Read the model definition and answer for the solid it produces. Units are mm, in the model's axes. Coordinates: 2 decimals unless noted, no trailing zeros. Loops run counter-clockwise (first coordinate to the right, second up) from the corner with the lowest first, then second, coordinate; pieces in that order, holes last.
Autodesk Inventor part; units mm, degrees
ref_plane "YZ Plane" through (0, 0, 0) normal (1, 0, 0) x (0, 1, 0)
ref_plane "XZ Plane" through (0, 0, 0) normal (0, 1, 0) x (-1, 0, 0)
ref_plane "XY Plane" through (0, 0, 0) normal (0, 0, 1) x (1, 0, 0)
sketch "Sketch1" plane through (0, 0, 0) normal (0, 0, 1) x (1, 0, 0)
  line L0 (95, 60) -> (105, 60)
  line L1 (105, 60) -> (105, 10)
  line L2 (105, 10) -> (100, 10)
  line L3 (100, 10) -> (100, 20)
  line L4 (100, 20) -> (95, 20)
  line L5 (95, 20) -> (95, 60)
  line L6 (105, -60) -> (95, -60)
  line L7 (95, -60) -> (95, -20)
  line L8 (95, -20) -> (100, -20)
  line L9 (100, -20) -> (100, -10)
  line L10 (100, -10) -> (105, -10)
  line L11 (105, -10) -> (105, -60)
  line L12 (120.5, 3.5) -> (123.5, 3.5)
  line L13 (123.5, 3.5) -> (123.5, 5)
  line L14 (123.5, 5) -> (127, 5)
  line L15 (127, 5) -> (127, -5)
  line L16 (127, -5) -> (123.5, -5)
  line L17 (123.5, -5) -> (123.5, -3.5)
  line L18 (123.5, -3.5) -> (120.5, -3.5)
  line L19 (120.5, -3.5) -> (120.5, -5)
  line L20 (120.5, -5) -> (117, -5)
  line L21 (117, -5) -> (117, -49)
  line L22 (117, -49) -> (107, -51)
  line L23 (107, -51) -> (107, -10)
  line L24 (107, -10) -> (112, -10)
  line L25 (112, -10) -> (112, -3.5)
  line L26 (112, -3.5) -> (100, -3.5)
  line L27 (100, -3.5) -> (100, -4)
  line L28 (100, -4) -> (45, -4)
  arc A0 (43, -6) -> (45, -4) centre (43, -4) ccw
  line L29 (43, -6) -> (42, -6)
  arc A1 (40, -4) -> (42, -6) centre (42, -4) ccw
  line L30 (40, -4) -> (5, -4)
  arc A2 (3, -6) -> (5, -4) centre (3, -4) ccw
  line L31 (3, -6) -> (2, -6)
  arc A3 (0, -4) -> (2, -6) centre (2, -4) ccw
  line L32 (0, -4) -> (0, 4)
  arc A4 (2, 6) -> (0, 4) centre (2, 4) ccw
  line L33 (2, 6) -> (3, 6)
  arc A5 (5, 4) -> (3, 6) centre (3, 4) ccw
  line L34 (5, 4) -> (40, 4)
  arc A6 (42, 6) -> (40, 4) centre (42, 4) ccw
  line L35 (42, 6) -> (43, 6)
  arc A7 (45, 4) -> (43, 6) centre (43, 4) ccw
  line L36 (45, 4) -> (100, 4)
  line L37 (100, 4) -> (100, 3.5)
  line L38 (100, 3.5) -> (112, 3.5)
  line L39 (112, 3.5) -> (112, 10)
  line L40 (112, 10) -> (107, 10)
  line L41 (107, 10) -> (107, 51)
  line L42 (107, 51) -> (117, 49)
  line L43 (117, 49) -> (117, 5)
  line L44 (117, 5) -> (120.5, 5)
  line L45 (120.5, 5) -> (120.5, 3.5)
  line L46 (92, 27.5) -> (92, 26)
  line L47 (92, 26) -> (42, 26)
  line L48 (42, 26) -> (42, 27.5)
  line L49 (42, 27.5) -> (92, 27.5)
  line L50 (92, -24) -> (92, -25.5)
  line L51 (92, -25.5) -> (42, -25.5)
  line L52 (42, -25.5) -> (42, -24)
  line L53 (42, -24) -> (92, -24)
  line L54 (92, -25.5) -> (82, -25.5)
  line L55 (82, -25.5) -> (82, -24)
  line L56 (82, -24) -> (77, -24)
  line L57 (77, -24) -> (77, -25.5)
  line L58 (77, -25.5) -> (57, -25.5)
  line L59 (57, -25.5) -> (57, -24)
  line L60 (57, -24) -> (52, -24)
  line L61 (52, -24) -> (52, -25.5)
  line L62 (52, -25.5) -> (42, -25.5)
  line L63 (42, -25.5) -> (42, 27.5)
  line L64 (92, 27.5) -> (92, 97.5)
  line L65 (92, -25.5) -> (92, -65.5)
  line L66 (92, -65.5) -> (132, -65.5)
  line L67 (132, -65.5) -> (142, -65.5)
  line L68 (132, -65.5) -> (132, 97.5)
  line L69 (142, -65.5) -> (142, 109.5)
  line L70 (42, 27.5) -> (34, 27.5)
  line L71 (95, 60) -> (105, 60)
  line L72 (105, 60) -> (105, 84)
  line L73 (105, 84) -> (95, 84)
  line L74 (95, 84) -> (95, 60)
  line L75 (95, 60) -> (95, 90)
  line L76 (95, 90) -> (132, 90)
  line L77 (95, 90) -> (92, 90)
  line L78 (142, -65.5) -> (142, -95.5)
  line L79 (142, -95.5) -> (92, -95.5)
  line L80 (92, -95.5) -> (34, -25.5)
  line L81 (34, -25.5) -> (34, 27.5)
  line L82 (0, 0) -> (71, 0)
  line L83 (23.8389, -219.7015) -> (66.8389, -219.7015)
  line L84 (66.8389, -219.7015) -> (66.8389, -198.7015)
  line L85 (66.8389, -198.7015) -> (23.8389, -198.7015)
  line L86 (23.8389, -198.7015) -> (23.8389, -219.7015)
  line L87 (45.3389, -198.7015) -> (45.3389, -219.7015)
  line L88 (66.8389, -198.7015) -> (66.8389, -203.7015)
  line L89 (66.8389, -203.7015) -> (70.8389, -203.7015)
  line L90 (70.8389, -203.7015) -> (70.8389, -213.7015)
  circle A8 centre (70.8389, -213.7015) radius 2
  circle A9 centre (70.8389, -203.7015) radius 2
  line L91 (66.8389, -209.2015) -> (56.8389, -209.2015)
  line L92 (56.8389, -209.2015) -> (56.8389, -189.2015)
  line L93 (56.8389, -189.2015) -> (56.8389, -229.2015)
  circle A10 centre (19.8389, -213.7015) radius 2
  circle A11 centre (19.8389, -203.7015) radius 2
  line L94 (33.8389, -189.2015) -> (33.8389, -229.2015)
  line L95 (42, -24) -> (83, -24)
  line L96 (83, -24) -> (83, -4)
  line L97 (83, -4) -> (42, -4)
  line L98 (42, -4) -> (42, -24)
  line L99 (62.5, -4) -> (62.5, -24)
  line L100 (83, -4) -> (83, -9)
  line L101 (83, -9) -> (87, -9)
  line L102 (87, -9) -> (87, -19)
  circle A12 centre (87, -9) radius 2
  circle A13 centre (87, -19) radius 2
  circle A14 centre (38, -9) radius 2
  circle A15 centre (38, -19) radius 2
  line L103 (92, -24) -> (92, 26)
  line L104 (109.5, -120.7576) -> (69.5, -120.7576)
  line L105 (69.5, -120.7576) -> (69.5, 125.4146)
  line L106 (142, 109.5) -> (67, 109.5)
  line L107 (67, 109.5) -> (67, 109.5)
  line L108 (67, 109.5) -> (34, 27.5)
  line L109 (34, 27.5) -> (69.5, 27.5)
  line L110 (69.5, 27.5) -> (69.5, 52.5)
  line L111 (92, 27.5) -> (69.5, 27.5)
  line L112 (92, 27.5) -> (77, 27.5)
  line L113 (77, 27.5) -> (77, 52.5)
  line L114 (77, 52.5) -> (78.5, 52.5)
  line L115 (78.5, 72.5) -> (77, 72.5)
  line L116 (77, 72.5) -> (77, 52.5)
  line L117 (78.5, 52.5) -> (81, 52.5)
  line L118 (81, 52.5) -> (81, 72.5)
  line L119 (81, 72.5) -> (78.5, 72.5)
  line L120 (81, 62.5) -> (79, 62.5)
  line L121 (79, 62.5) -> (74, 62.5)
  line L122 (74, 62.5) -> (84, 62.5)
  circle A16 centre (74, 62.5) radius 1.5
  circle A17 centre (84, 62.5) radius 1.5
  line L123 (92, -95.5) -> (92, -90.5)
  line L124 (92, -90.5) -> (97, -90.5)
  line L125 (97, -90.5) -> (117, -90.5)
  line L126 (117, -90.5) -> (117, -89)
  line L127 (117, -89) -> (97, -89)
  line L128 (97, -89) -> (97, -90.5)
  line L129 (97, -89) -> (97, -79)
  line L130 (97, -79) -> (117, -79)
  line L131 (117, -79) -> (117, -77.5)
  line L132 (117, -77.5) -> (97, -77.5)
  line L133 (97, -77.5) -> (97, -79)
  line L134 (107, -90.5) -> (107, -84)
  circle A18 centre (107, -84) radius 1.5
  point P0 (59.5188, -93.2152)
  point P1 (83, -4)
  point P2 (83, -24)
  dimension "d0" = 10
  dimension "d1" = 1.5
  dimension "d2" = 5
  dimension "d3" = 1.5
  dimension "d4" = 20
  dimension "d5" = 1.5
  dimension "d6" = 5
  dimension "d7" = 1.5
  dimension "d8" = 70
  dimension "d9" = 40
  dimension "d10" = 40
  dimension "d11" = 40
  dimension "d12" = 10
  dimension "d13" = 175
  dimension "d14" = 8
  dimension "d15" = 10
  dimension "d16" = 24
  dimension "d17" = 30
  dimension "d19" = 30
  dimension "d20" = 50
  dimension "d21" = 71
  dimension "d22" = 43
  dimension "d23" = 21
  dimension "d24" = 5
  dimension "d25" = 4
  dimension "d26" = 10
  dimension "d27" = 4
  dimension "d28" = 4
  dimension "d29" = 10
  dimension "d30" = 20
  dimension "d31" = 40
  dimension "d32" = 41
  dimension "d33" = 20
  dimension "d34" = 5
  dimension "d35" = 4
  dimension "d36" = 10
  dimension "d37" = 4
  dimension "d38" = 4
  dimension "d48" = 40
  dimension "d49" = 3
  dimension "d50" = 75
  dimension "d51" = 0
  dimension "d62" = 15
  dimension "d63" = 25
  dimension "d64" = 1.5
  dimension "d65" = 20
  dimension "d73" = 2.5
  dimension "d74" = 2
  dimension "d75" = 5
  dimension "d76" = 10
  dimension "d77" = 3
  dimension "d78" = 3
  dimension "d81" = 5
  dimension "d82" = 5
  dimension "d83" = 20
  dimension "d84" = 1.5
  dimension "d85" = 10
  dimension "d86" = 20
  dimension "d87" = 1.5
  dimension "d88" = 3
extrude "Extrusion1" add sketch "Sketch1" along normal blind 1.5 contours A16 | A17 | L116 L121 L120 L118 L117 L114 | L77 L64 L49 L105 L106 L69 L67 L68 L76 | L133 L132 L131 L130 | A18 | L128 L127 L134 L125 | L67 L78 L79 L80 L105 L51 L65 L66 | L103 L36 L105 L47 | L105 L36 A7 L35 L63 L47 | L103 L28 L105 L36 | L49 L70 L108 L106 L105 | L53 L96 L28 L103 | L63 A6 L34 L81 L70 L48 | L105 L82 L63 L35 A7 L36 | L116 L115 L119 L118 L120 L121 | L80 L81 L30 A1 L63 L52 L51 L105 | L63 L82 L81 L34 A6 | L105 L28 L97 L63 L82 | L63 A1 L30 L81 L82 | L134 L127 L126 L125
sketch "Sketch2" plane through (0, 0, 1.5) normal (0, 0, 1) x (1, 0, 0)
  line L0 (42, 26) -> (42, 27.5)
  line L1 (42, 26.75) -> (62, 26.75)
  line L2 (62, 26.75) -> (62, 31.75)
  line L3 (62, 31.75) -> (62, 21.75)
  circle A0 centre (62, 31.75) radius 1.5
  circle A1 centre (62, 21.75) radius 1.5
  point P0 (0, 0)
  dimension "d41" = 20
  dimension "d42" = 5
  dimension "d43" = 10
  dimension "d44" = 3
  dimension "d45" = 3
extrude "Extrusion2" cut sketch "Sketch2" against normal blind 1.5
extrude "Extrusion5" cut sketch "Sketch1" along normal blind 1.5 contours A16 | A17 | L116 L121 L120 L118 L117 L114 | L116 L115 L119 L118 L120 L121
extrude "Extrusion6" cut sketch "Sketch1" along normal blind 1.5 contours L133 L132 L131 L130 | A18 | L128 L127 L134 L125 | L134 L127 L126 L125
sketch "Sketch3" plane through (0, 0, 1.5) normal (0, 0, 1) x (1, 0, 0)
  line L0 (81, 72.5) -> (81, 52.5)
  line L1 (81, 72.5) -> (81, 102.5)
  line L2 (42, 27.5) -> (92, 27.5)
  line L3 (81, 102.5) -> (81, 92.5)
  line L4 (81, 102.5) -> (83.5, 102.5)
  line L5 (83.5, 102.5) -> (83.5, 92.5)
  line L6 (83.5, 102.5) -> (88.5, 102.5)
  line L7 (88.5, 102.5) -> (88.5, 101)
  line L8 (88.5, 101) -> (83.5, 101)
  line L9 (83.5, 101) -> (83.5, 102.5)
  line L10 (83.5, 92.5) -> (88.5, 92.5)
  line L11 (88.5, 92.5) -> (88.5, 91)
  line L12 (88.5, 91) -> (83.5, 91)
  line L13 (83.5, 91) -> (83.5, 92.5)
  point P0 (0, 0)
  dimension "d93" = 30
  dimension "d94" = 10
  dimension "d95" = 2.5
  dimension "d96" = 5
  dimension "d97" = 1.5
  dimension "d98" = 5
  dimension "d99" = 1.5
extrude "Extrusion7" cut sketch "Sketch3" against normal blind 1.5
sketch "Sketch4" plane through (0, 0, 1.5) normal (0, 0, 1) x (1, 0, 0)
  line L0 (142, -95.5) -> (142, 109.5)
  line L1 (142, 109.5) -> (142, 99.5)
  line L2 (142, 99.5) -> (132, 99.5)
  line L3 (132, 99.5) -> (127, 99.5)
  circle A0 centre (127, 99.5) radius 1.5
  circle A1 centre (134.5, 95.1699) radius 1.5
  circle A2 centre (134.5, 103.8301) radius 1.5
  line L4 (142, -95.5) -> (142, -85.5)
  line L5 (142, -85.5) -> (132, -85.5)
  line L6 (132, -85.5) -> (127, -85.5)
  circle A3 centre (127, -85.5) radius 1.5
  circle A4 centre (134.5, -89.8301) radius 1.5
  circle A5 centre (134.5, -81.1699) radius 1.5
  point P0 (0, 0)
  dimension "d102" = 10
  dimension "d103" = 10
  dimension "d104" = 5
  dimension "d105" = 3
  dimension "d108" = 360
  dimension "d110" = 10
  dimension "d111" = 10
  dimension "d112" = 5
  dimension "d113" = 3
  dimension "d116" = 360
extrude "Extrusion8" cut sketch "Sketch4" against normal blind 1.5
properties part number "SIdeFinal"
Item 1: A cutting plane is placed at C-C on y = -19. Determine the outline of the cut face in (x, z).
Numbers:
outline: (34, 0) - (36, 0) - (36, 1.5) - (34, 1.5) - close; (40, 0) - (42, 0) - (42, 1.5) - (40, 1.5) - close; (83, 0) - (85, 0) - (85, 1.5) - (83, 1.5) - close; (89, 0) - (92, 0) - (92, 1.5) - (89, 1.5) - close; (132, 0) - (142, 0) - (142, 1.5) - (132, 1.5) - close
Item 2: Determine the mould class of faces 1 (the face through (87, 8, 1.5)), 2 (the face through (50.73, 69.07, 0.74)), 3 (the face through (88.908, -19.601, 0.74)) for opening direction X: released by +X, released by -X, zero draft, split by the parting line, or undercut.
Numbers:
face 1: zero draft
face 2: released by -X
face 3: undercut
Item 3: A cutting plane is placed at B-B on x = 113.5. Determine the outline of the cut face in (y, z).
Numbers:
outline: (-95.5, 0) - (-90.5, 0) - (-90.5, 1.5) - (-95.5, 1.5) - close; (-89, 0) - (-79, 0) - (-79, 1.5) - (-89, 1.5) - close; (-77.5, 0) - (-65.5, 0) - (-65.5, 1.5) - (-77.5, 1.5) - close; (90, 0) - (109.5, 0) - (109.5, 1.5) - (90, 1.5) - close
Item 4: A cutting plane is placed at D-D on x = 79. Determine the outline of the cut face in (y, z), then the cut area to 3 significant figures.
Numbers:
outline: (-79.81, 0) - (-25.5, 0) - (-25.5, 1.5) - (-79.81, 1.5) - close; (-4, 0) - (26, 0) - (26, 1.5) - (-4, 1.5) - close; (27.5, 0) - (52.5, 0) - (52.5, 1.5) - (27.5, 1.5) - close; (72.5, 0) - (109.5, 0) - (109.5, 1.5) - (72.5, 1.5) - close
area: 219 mm2
Item 5: A cutting plane is placed at A-A on y = 6. Determine the outline of the cut face in (x, z), then the cut area to 3 significant figures.
Numbers:
outline: (34, 0) - (92, 0) - (92, 1.5) - (34, 1.5) - close; (132, 0) - (142, 0) - (142, 1.5) - (132, 1.5) - close
area: 102 mm2
Item 6: Find the intervals of material crossed by line 1 along Y through (x, z) = (134.5, 1); line 2 along Y through (x, z) = (107, 0.75); line 3 along Y through (x, z) = (112, 1.1), in increasing order.
Numbers:
line 1: y = -95.5 to -91.33, -88.33 to -82.67, -79.67 to 93.67, 96.67 to 102.33, 105.33 to 109.5
line 2: y = -95.5 to -90.5, -89 to -85.5, -82.5 to -79, -77.5 to -65.5, 90 to 109.5
line 3: y = -95.5 to -90.5, -89 to -79, -77.5 to -65.5, 90 to 109.5
